Work out the finished part from the listing and answer in its coordinate system (mm). Give positions to 0.01 mm unless a question says otherwise; leave off trailing zeros. Order: outer loops, then holes, each group sorted by start corner. A loop starts at its lowest first (then second) coordinate and runs counter-clockwise, first axis right, second up. Notation, with made-up numbers: (-19.5, 14.5) - (6.5, 14.5) arc R22 cw to (6.5, 35.5) - close; hole circle Ø9 at (-5, 44). An arc over 180 degrees is marked (long way). Write each question's results on one line, items separated by ' | '.
from build123d import *

# Parameters (mm, degrees)
BOSS_EXTRUDE1_DEPTH = 1
SKETCH2_R           = 0.3175
BOSS_EXTRUDE2_DEPTH = 0.127


with BuildPart() as part:
    # Sketch1 → Boss-Extrude1 (new body)
    with BuildSketch(Plane(origin=(0, 0, 0), x_dir=(1, 0, 0), z_dir=(0, 1, 0))):
        with BuildLine():
            Line((-12.46, 7.5), (15, 7.5))
            Line((15, 7.5), (15, -4.96))
            Line((15, -4.96), (14.667795167, -4.96))
            ThreePointArc((14.667795167, -4.96), (12.312776928, -4.866304174), (12.46, -7.218582895))
            Line((12.46, -7.218582895), (12.46, -7.5))
            Line((12.46, -7.5), (-15, -7.5))
            Line((-15, -7.5), (-15, 4.96))
            Line((-15, 4.96), (-14.707321343, 4.96))
            ThreePointArc((-14.707321343, 4.96), (-12.359897737, 4.833074853), (-12.46, 7.181795167))
            Line((-12.46, 7.181795167), (-12.46, 7.5))
        make_face()
    extrude(amount=BOSS_EXTRUDE1_DEPTH)

    # Sketch2 → Boss-Extrude2 (add)
    with BuildSketch(Plane(origin=(0, 1, 0), x_dir=(1, 0, 0), z_dir=(0, 1, 0))):
        with Locations(Location((-9.92, 2.025, 0), (0, 0, 270))):
            Circle(SKETCH2_R)
        with Locations(Location((-5.094, -0.388, 0), (0, 0, 270))):
            Circle(SKETCH2_R)
        with Locations(Location((-6.11, -2.166, 0), (0, 0, 270))):
            Circle(SKETCH2_R)
        with Locations(Location((-0.522, 2.66, 0), (0, 0, 270))):
            Circle(SKETCH2_R)
        with Locations(Location((-0.014, -0.515, 0), (0, 0, 270))):
            Circle(SKETCH2_R)
    extrude(amount=BOSS_EXTRUDE2_DEPTH)


solid = part.part
1. A cutting plane is placed at D-D, the plane x = 11. Write down the section's boundary in (y, z), then the cut area to 3 significant figures.
Answer list:
outline: (0, -7.5) - (1, -7.5) - (1, 7.5) - (0, 7.5) - close | area: 15.0 mm^2
2. Straight lines are drawn through the part: line 1 (Y direction, x = -9.25, z = 4.5); line 2 (X direction, y = 0.4, z = 7.25); line 3 (Z direction, x = -5, y = 1.05). For each, find the intervals that lie inside material, in ascending order. Write a range as [from, to].
Answer list:
line 1: [0, 1] | line 2: [-15, 12.46] | line 3: [0.08, 0.69]
3. A cutting plane is placed at C-C, the plane x = -6.11. Write down the section's boundary in (y, z), then the cut area to 3 significant figures.
Answer list:
outline: (0, -7.5) - (1, -7.5) - (1, 1.85) - (1.13, 1.85) - (1.13, 2.48) - (1, 2.48) - (1, 7.5) - (0, 7.5) - close | area: 15.1 mm^2
4. Given P1, Ø5, axis at x = 9, z = 1, coming from the +Y side; P2, Ø2.5, axis at x = -13.476, z = -5.962, coming from the +Y side, each flat-ended and moving along its own axis, determine where each tip first touches the part or whether it passes through.
Answer list:
P1: y = 1 | P2: through
5. A cutting plane is placed at B-B, the plane z = -2.66. Write down the section's boundary in (x, y).
Answer list:
outline: (-15, 0) - (15, 0) - (15, 1) - (-0.2, 1) - (-0.2, 1.13) - (-0.84, 1.13) - (-0.84, 1) - (-15, 1) - close
6. Determine the mould class of faces 1 (the face through (15, 0.5, -1.4)), 2 (the face through (-1.1, 0.5, 7.5)), 3 (the face through (12.34, 0.49, 4.84)), 4 (the face through (-12.387, 0.493, -4.807)) for opening direction X: +X half, -X half, draft (parallel to the pull), parting line (faces both ways), or undercut.
Answer list:
face 1: +X half | face 2: draft | face 3: undercut | face 4: undercut
